from build123d import *

# Parameters (mm, degrees)
ESQUISSE1_W        = 20.2
ESQUISSE1_H        = 40.2
BOSS_EXTRU_1_DEPTH = 15


with BuildPart() as part:
    # Esquisse1 → Boss.-Extru.1 (new body)
    with BuildSketch(Plane.XY):
        with BuildLine():
            Line((-35.249311761, -55), (-35.249311761, -75))
            Line((-35.249311761, -75), (38.140688239, -75))
            Line((38.140688239, -75), (38.140688239, -55))
            Line((38.140688239, -55), (53.140688239, -55))
            Line((53.140688239, -55), (53.140688239, 5))
            Line((53.140688239, 5), (38.140688239, 5))
            Line((38.140688239, 5), (38.140688239, 25))
            Line((38.140688239, 25), (53.140688239, 25))
            Line((53.140688239, 25), (53.140688239, 73.326682602))
            ThreePointArc((53.140688239, 73.326682602), (1.445688239, 125.021682602), (-50.249311761, 73.326682602))
            Line((-50.249311761, 73.326682602), (-50.249311761, 25))
            Line((-50.249311761, 25), (-35.249311761, 25))
            Line((-35.249311761, 25), (-35.249311761, 5))
            Line((-35.249311761, 5), (-50.249311761, 5))
            Line((-50.249311761, 5), (-50.249311761, -55))
            Line((-50.249311761, -55), (-35.249311761, -55))
        make_face()
        with Locations((1.445688239, 60.982767533)):
            Rectangle(ESQUISSE1_W, ESQUISSE1_H, mode=Mode.SUBTRACT)
    extrude(amount=BOSS_EXTRU_1_DEPTH)


solid = part.part
Source: CAD feature listing. Evaluate the final solid. Frame: model axes, mm. A direction names the side the tool comes from. Coordinates: 2 decimals unless noted, no trailing zeros. Order: outer loops, then holes, each group sorted by start corner. A loop starts at its lowest first (then second) coordinate and runs counter-clockwise, first axis right, second up.
Item 1: Pull-direction query (X, two-part tool) for faces 1 (the face through (1, 81.083, 7)), 2 (the face through (46, 25, 7)), 3 (the face through (-50.249, 50, 7)); classes: pulls with the +X half, pulls with the -X half, needs draft (parallel to the pull), parting line crosses it, or undercut.
Output values:
face 1: undercut
face 2: needs draft
face 3: pulls with the -X half
Item 2: Cut plane C-C (y = 15.5). Return loops of the section in (x, z).
Output values:
outline: (-35.25, 0) - (38.14, 0) - (38.14, 15) - (-35.25, 15) - close
Item 3: Cut plane B-B (x = 8.5). Return loops of the section in (y, z).
Output values:
outline: (-75, 0) - (40.88, 0) - (40.88, 15) - (-75, 15) - close; (81.08, 0) - (124.54, 0) - (124.54, 15) - (81.08, 15) - close
Item 4: Cut plane D-D (x = -41). Return loops of the section in (y, z), plus the area to 3 significant figures.
Output values:
outline: (-55, 0) - (5, 0) - (5, 15) - (-55, 15) - close; (25, 0) - (102.83, 0) - (102.83, 15) - (25, 15) - close
area: 2,070 mm2
Item 5: Material intervals for line 1 (Y direction, x = -0.5, z = 10.5); line 2 (X direction, y = -61, z = 14); line 3 (Y direction, x = -41.5, z = 9.75), sorted ascending.
Output values:
line 1: y = -75 to 40.88, 81.08 to 124.99
line 2: x = -35.25 to 38.14
line 3: y = -55 to 5, 25 to 102.1
Item 6: Set-up query: faces 4 (the face through (46, -55, 7)), 5 (the face through (11.546, 61, 7)), 6 (the face through (-35.249, 15, 7)). Return all of +Z, -Z, +X, -X, +Y, -Y with unobstructed straight access to the full face (end or side cutting, diameter ignored); none if empty.
Output values:
face 4: +Z, -Z, +X, -Y
face 5: +Z, -Z
face 6: +Z, -Z, -X
Item 7: First-contact query: P1, Ø4.5, axis at y = 15.5, z = 8.5, coming from the +X side; P2, Ø4.5, axis at x = 48, z = 4.5, coming from the -Y side; P3, Ø6, axis at x = 34, z = 4, coming from the +Y side. Flat tips, straight axial feed; report the tip coordinate or a pass-through.
Output values:
P1: stops at x = 38.14
P2: stops at y = -55
P3: stops at y = 115.74
Item 8: Cut plane A-A (z = 4.75). Return loops of the section in (x, y) (3 decimals).
Output values:
outline: (-50.249, -55) - (-35.249, -55) - (-35.249, -75) - (38.141, -75) - (38.141, -55) - (53.141, -55) - (53.141, 5) - (38.141, 5) - (38.141, 25) - (53.141, 25) - (53.141, 73.327) arc R51.695 ccw to (-50.249, 73.327) - (-50.249, 25) - (-35.249, 25) - (-35.249, 5) - (-50.249, 5) - close; hole (-8.654, 40.883) - (11.546, 40.883) - (11.546, 81.083) - (-8.654, 81.083) - close
